```python
from build123d import *

# Parameters (mm, degrees)
F0_W     = 72.5
F0_H     = 46
F0_R     = 4.5
F1_DEPTH = 3
F2_DEPTH = 8
F3_D     = 3.3
F4_W     = 9
F4_H     = 8
F5_DEPTH = 5
F6_W     = 9.5978157372
F6_H     = 8
F7_DEPTH = 5


with BuildPart() as f1:
    # F0 (on Top) → F1 (new body)
    with BuildSketch(Plane.XY):
        Rectangle(F0_W, F0_H)
        with Locations((-23.75, -10.5)):
            Circle(F0_R, mode=Mode.SUBTRACT)
        with Locations((21.5, -10.5)):
            Circle(F0_R, mode=Mode.SUBTRACT)
        with Locations((-23.75, -10.5)):
            Circle(F0_R)
        with Locations((21.5, -10.5)):
            Circle(F0_R)
    extrude(amount=F1_DEPTH)

    # F0 (on Top) → F2 (join)
    with BuildSketch(Plane.XY):
        with Locations((-23.75, -10.5)):
            Circle(F0_R)
        with Locations((21.5, -10.5)):
            Circle(F0_R)
    extrude(amount=F2_DEPTH)

    # F3 (through all)
    with Locations(Plane(origin=(0, 0, 0), x_dir=(1, 0, 0), z_dir=(0, 0, -1))):
        with Locations((21.5, 10.5), (-23.75, 10.5)):
            Hole(F3_D / 2)

    # F4 (on face) → F5 (join)
    with BuildSketch(Plane.XY.offset(3)):
        with Locations((-23.75, 13.5)):
            Rectangle(F4_W, F4_H)
    extrude(amount=F5_DEPTH)

    # F6 (on face) → F7 (join)
    with BuildSketch(Plane.XY.offset(3)):
        with Locations((21.0489078686, 13.5)):
            Rectangle(F6_W, F6_H)
    extrude(amount=F7_DEPTH)


solid = f1.part
```
For this review, take the finished solid that the model builds, in its own axes (mm). A direction names the side the tool comes from. Give positions to 0.01 mm unless a question says otherwise; leave off trailing zeros. Write each loop counter-clockwise with the first axis right and the second up, starting at its lowest first coordinate (ties: lowest second). Pieces come first, ordered by that corner, then holes. Notation, with made-up numbers: M 21.5,50.25 L 67.5,50.25 A28 cw 67.5,85.25 Z; hole C 71.25,24 d1. An arc over 180 degrees is marked long. Answer as a JSON object with one key per item and string values. Group by question number.
Item 1: For pin 1 Ø2.5 at (x, z) = (-25.5, 6.5) entering from +Y; pin 2 Ø4 at (x, z) = (-21.5, 5.5) entering from -Y; pin 3 Ø3 at (y, z) = (-7, 5) entering from +X, all flat-tipped, find the tip position at first contact; note any pin that passes through.
Item 2: For probe 1 along X at (y, z) = (-10.5, 3.5); probe 2 along X at (y, z) = (-10.5, 1.75); probe 3 along Y at (x, z) = (21.5, 2.75), list the stretches that pass through material, from the lowest coordinate up. Write a range as [from, to].
Item 3: Consider section D-D on y = -1. Write out the cut boundary in (x, z).
Item 4: Draft analysis for pull direction X (two halves, no side actions). For faces 6 (the flat face through (-28.25, 13, 5)), 7 (the flat face through (-23.8, -12.4, 8)), 8 (the cylindrical face through (-28.246, -10.302, 5.465)), state which applies: +X half, -X half, draft (parallel to the pull), parting line (faces both ways), or undercut.
Item 5: Consider section C-C on y = -10.5. Write out the cut boundary in (x, z), plus the area to 3 significant figures.
Item 6: Consider section A-A on x = 21.5. Write out the cut boundary in (y, z).
Item 7: Tool access review of faces 1 (the flat face through (16.25, 13, 5)), 2 (the flat face through (-24, 17.5, 5)), 3 (the cylindrical face through (17.004, -10.302, 5.465)), 4 (the flat face through (25.848, 13, 5)), 5 (the flat face through (21, 9.5, 5)): name each direction out of +Z, -Z, +X, -X, +Y, -Y from which nothing blocks a thin tool from reaching the whole face with its end or side.
Item 8: Consider section B-B on z = 6.5. Write out the cut boundary in (x, y), plus the area to 3 significant figures.
Check result:
{
 "1": {"pin 1": "stops at y = 17.5", "pin 2": "stops at y = -14.99", "pin 3": "stops at x = 25.53"},
 "2": {"probe 1": "x = [-28.25, -25.4], [-22.1, -19.25], [17, 19.85], [23.15, 26]", "probe 2": "x = [-36.25, -25.4], [-22.1, 19.85], [23.15, 36.25]", "probe 3": "y = [-23, -12.15], [-8.85, 23]"},
 "3": {"outline": "M -36.25,0 L 36.25,0 L 36.25,3 L -36.25,3 Z"},
 "4": {"face 6": "-X half", "face 7": "draft", "face 8": "undercut"},
 "5": {"outline": "M -36.25,0 L -25.4,0 L -25.4,8 L -28.25,8 L -28.25,3 L -36.25,3 Z; M -22.1,0 L 19.85,0 L 19.85,8 L 17,8 L 17,3 L -19.25,3 L -19.25,8 L -22.1,8 Z; M 23.15,0 L 36.25,0 L 36.25,3 L 26,3 L 26,8 L 23.15,8 Z", "area": "255 mm^2"},
 "6": {"outline": "M -23,0 L -12.15,0 L -12.15,8 L -15,8 L -15,3 L -23,3 Z; M -8.85,0 L 23,0 L 23,3 L 17.5,3 L 17.5,8 L 9.5,8 L 9.5,3 L -6,3 L -6,8 L -8.85,8 Z"},
 "7": {"face 1": "+Z, +Y, -Y", "face 2": "+Z, +X, -X, +Y", "face 3": "+Z", "face 4": "+Z, +X, +Y", "face 5": "+Z, +X, -X"},
 "8": {"outline": "C -23.75,-10.5 d9; M -28.25,9.5 L -19.25,9.5 L -19.25,17.5 L -28.25,17.5 Z; M 16.25,9.5 L 25.85,9.5 L 25.85,17.5 L 16.25,17.5 Z; C 21.5,-10.5 d9; hole C -23.75,-10.5 d3.3; hole C 21.5,-10.5 d3.3", "area": "259 mm^2"}
}
